from build123d import *

# Parameters (mm, degrees)
F2_DEPTH = 3
F3_SIZE  = 0.4


with BuildPart() as f2:
    # F1 (on Top) → F2 (new body)
    with BuildSketch(Plane.XY):
        with BuildLine():
            ThreePointArc((0, 17), (16.4207390469, -4.3999237667), (-8.5, -14.7224318643))
            ThreePointArc((-8.5, -14.7224318643), (-10.5490381057, -15.27146997), (-10, -17.3205080757))
            ThreePointArc((-10, -17.3205080757), (19.3185165258, -5.1763809021), (0, 20))
            Line((0, 20), (-30, 20))
            ThreePointArc((-30, 20), (-33.380740392, 24.4058666579), (-28.25, 26.5310889132))
            ThreePointArc((-28.25, 26.5310889132), (-26.2009618943, 27.0801270189), (-26.75, 29.1291651246))
            ThreePointArc((-26.75, 29.1291651246), (-36.2785178709, 25.1823237932), (-30, 17))
            Line((-30, 17), (0, 17))
        make_face()
    extrude(amount=F2_DEPTH)

    # F3
    f3_edges = [f2.edges().sort_by_distance(p)[0] for p in [
        (-15, 17, 3),
        (-15, 17, 0),
    ]]
    chamfer(f3_edges, length=F3_SIZE)


solid = f2.part
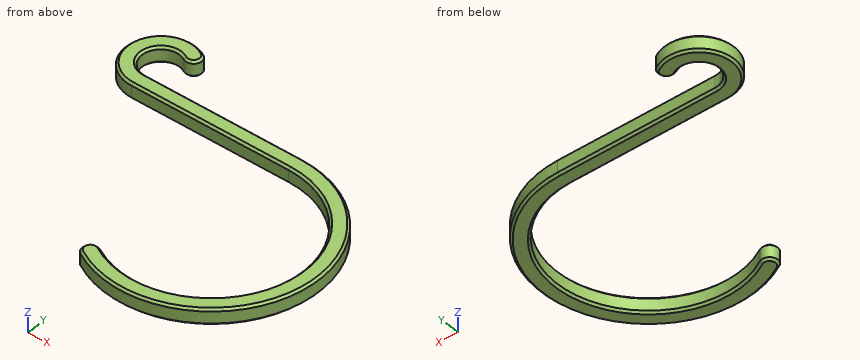
Could you check a few things on this model? Use its own coordinates, in mm. Coordinates: 2 decimals unless noted, no trailing zeros. Loops run counter-clockwise (first coordinate to the right, second up) from the corner with the lowest first, then second, coordinate; pieces in that order, holes last.
1. For P1, Ø4, axis at x = -30, y = 23.5, coming from the +Z side; P2, Ø1.5, axis at y = 6.5, z = 1, coming from the +X side; P3, Ø1.5, axis at x = -8, z = 1.5, coming from the +Y side; P4, Ø1, axis at x = 8.5, z = 1.5, coming from the -Y side, each with a flat end and sliding along its axis, tell me the tip position at first contact or that it passes through.
2. I need wall thicknesses on L1, parallel to Y at x = -30, z = 2.1; L2, parallel to X at y = 23.5, z = 1.05; L3, parallel to Y at x = -10, z = 2.7. Which ranges of each line are inside material? Lowest first, please.
3. Imagine slicing it at B-B (x = -14.5). Please give me the cut outline in (y, z), and give its area (3 significant figures).
4. Imagine slicing it at A-A (y = 23.5). Please give me the cut outline in (x, z).
Computed values:
1. P1: passes through
1. P2: stops at x = 19.16
1. P3: stops at y = 20
1. P4: stops at y = -18.33
2. L1: y = 17 to 20, 27 to 30
2. L2: x = -36.5 to -33.5
2. L3: y = -17.2 to -14.84, 17.1 to 19.9
3. outline: (17, 0.4) - (17.4, 0) - (19.6, 0) - (20, 0.4) - (20, 2.6) - (19.6, 3) - (17.4, 3) - (17, 2.6) - close
3. area: 8.68 mm2
4. outline: (-36.5, 0.4) - (-36.1, 0) - (-33.9, 0) - (-33.5, 0.4) - (-33.5, 2.6) - (-33.9, 3) - (-36.1, 3) - (-36.5, 2.6) - close
